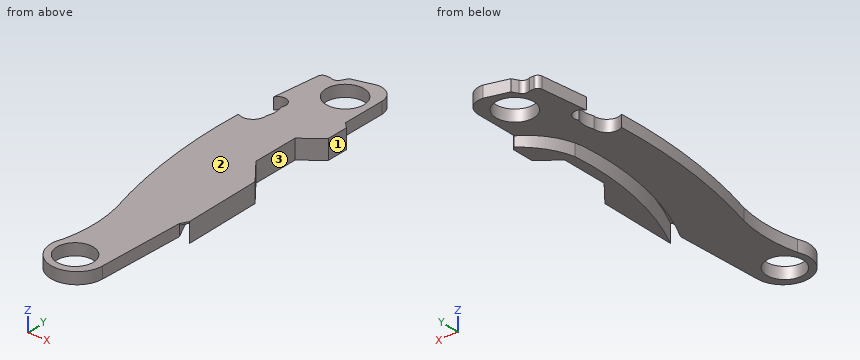
```python
from build123d import *

# Parameters (mm, degrees)
SKETCH1_R           = 3.1115
SKETCH1_R_2         = 2.9845
BOSS_EXTRUDE1_DEPTH = 1.905
CUT_EXTRUDE1_DEPTH  = 1.651
BOSS_EXTRUDE2_START = 1.27
BOSS_EXTRUDE2_DEPTH = 1.27
FILLET1_R           = 0.762
SCALE1_SCALE        = 1.0350841


with BuildPart() as part:
    # Sketch1 → Boss-Extrude1 (new body)
    with BuildSketch(Plane.XY):
        with BuildLine():
            Line((11.455137598, 2.171678291), (10.988691825, -12.194362723))
            ThreePointArc((10.988691825, -12.194362723), (5.753403312, -16.215064409), (2.835732355, -10.293790556))
            ThreePointArc((2.835732355, -10.293790556), (3.433990562, -5.092237988), (2.835732355, 0.109314579))
            ThreePointArc((2.835732355, 0.109314579), (-0.031028462, 13.845472924), (-0.62536344, 27.864999648))
            ThreePointArc((-0.62536344, 27.864999648), (1.430712022, 27.922734075), (2.296539191, 29.788510826))
            ThreePointArc((2.296539191, 29.788510826), (2.577489408, 31.240527695), (2.296539191, 32.692544565))
            ThreePointArc((2.296539191, 32.692544565), (1.793167017, 34.551137871), (-0.054485013, 34.008980516))
            Line((-0.054485013, 34.008980516), (0.8585336, 42.2777508))
            Line((0.8585336, 42.2777508), (2.296539191, 42.2777508))
            ThreePointArc((2.296539191, 42.2777508), (3.056005554, 42.188646363), (3.657600202, 42.660676697))
            Line((3.657600202, 42.660676697), (4.193229273, 43.60832813))
            Line((4.193229273, 43.60832813), (7.858351578, 44.652580854))
            ThreePointArc((7.858351578, 44.652580854), (10.042305559, 44.016121117), (10.988691825, 41.94752521))
            Line((10.988691825, 41.94752521), (10.988691825, 34.921067581))
            Line((10.988691825, 34.921067581), (11.90077889, 34.008980516))
            Line((11.90077889, 34.008980516), (11.90077889, 30.495455397))
            Line((11.90077889, 30.495455397), (8.673783219, 27.864999648))
            Line((8.673783219, 27.864999648), (8.673783219, 20.285030353))
            Line((8.673783219, 20.285030353), (11.90077889, 16.326210266))
            Line((11.90077889, 16.326210266), (12.102967643, 3.372738413))
            Line((12.102967643, 3.372738413), (11.455137598, 2.171678291))
        make_face()
        with Locations(Location((6.72245078, 39.860230894, 0), (0, 0, 180))):
            Circle(SKETCH1_R, mode=Mode.SUBTRACT)
        with Locations(Location((6.525698673, -12.20338788, 0), (0, 0, 180))):
            Circle(SKETCH1_R_2, mode=Mode.SUBTRACT)
    extrude(amount=BOSS_EXTRUDE1_DEPTH)

    # Sketch7 → Cut-Extrude1 (cut)
    with BuildSketch(Plane(origin=(0, 0, 0), x_dir=(-1, 0, 0), z_dir=(0, 0, -1))):
        with BuildLine():
            Line((-12.102967643, 3.372738413), (-11.455137598, 2.171678291))
            ThreePointArc((-11.455137598, 2.171678291), (-6.980280612, 14.413742368), (-6.117233468, 27.41941911))
            ThreePointArc((-6.117233468, 27.41941911), (-7.707175586, 31.719484817), (-10.988691825, 34.921067581))
            Line((-10.988691825, 34.921067581), (-11.444735357, 34.465024049))
            ThreePointArc((-11.444735357, 34.465024049), (-8.702145747, 31.480644967), (-7.139396786, 27.740841235))
            ThreePointArc((-7.139396786, 27.740841235), (-7.956577994, 15.217724405), (-12.102967643, 3.372738413))
        make_face()
    extrude(amount=-CUT_EXTRUDE1_DEPTH, mode=Mode.SUBTRACT)

    # Sketch8 → Boss-Extrude2 (add)
    with BuildSketch(Plane(origin=(0, 0, 0), x_dir=(-1, 0, 0), z_dir=(0, 0, -1)).offset(BOSS_EXTRUDE2_START)):
        with BuildLine():
            Line((-11.90077889, 16.326210266), (-12.102967643, 3.372738413))
            ThreePointArc((-12.102967643, 3.372738413), (-7.956577994, 15.217724405), (-7.139396786, 27.740841235))
            ThreePointArc((-7.139396786, 27.740841235), (-8.702145747, 31.480644967), (-11.444735357, 34.465024049))
            Line((-11.444735357, 34.465024049), (-11.90077889, 34.008980516))
            Line((-11.90077889, 34.008980516), (-11.90077889, 30.495455397))
            Line((-11.90077889, 30.495455397), (-8.673783219, 27.864999648))
            Line((-8.673783219, 27.864999648), (-8.673783219, 20.285030353))
            Line((-8.673783219, 20.285030353), (-11.90077889, 16.326210266))
        make_face()
    extrude(amount=-BOSS_EXTRUDE2_DEPTH)

    # Fillet1
    fillet1_edges = [part.edges().sort_by_distance(p)[0] for p in [
        (0.8585336, 42.2777508, 0.9525),
    ]]
    fillet(fillet1_edges, radius=FILLET1_R)


with BuildPart() as part_1:
    # Scale1: scaled about (6.266812803, 15.225745721, 0.817427893)
    add(part.part.scale(SCALE1_SCALE).moved(Location((-0.219865487, -0.534181585, -0.028678722))))


solid = part_1.part
```
Work out the finished part from the listing and answer in its coordinate system (mm). Face numbers are marked on the shaded views. A direction names the side the tool comes from. Give positions to 0.01 mm unless a question says otherwise; leave off trailing zeros. Order: outer loops, then holes, each group sorted by start corner. A loop starts at its lowest first (then second) coordinate and runs counter-clockwise, first axis right, second up. Notation, with made-up numbers: (34, 18.5) -> (69, 18.5) arc R20 cw to (69, 25.5) -> close; hole circle Ø9 at (-33.5, 6.5). An arc over 180 degrees is marked (long way). Answer as CSV lines item,"result". Start each with the question number.
(1) Section A-A, the plane z = 0.95 is taken. Write down the section's boundary in (x, y) (1 decimal).
(2) Section B-B, the plane x = 5 is taken. Write down the section's boundary in (y, z).
(3) Consider line 1 along Y through (x, z) = (4.5, 1.85); line 2 along X through (y, z) = (24.5, 1.65); line 3 along Y through (x, z) = (5.75, 1.85). Determine where each line is inside the solid, lowest interval first.
(4) Section D-D, the plane y = 4.5 is taken. Write down the section's boundary in (x, z).
(5) Section C-C, the plane y = 41.5 is taken. Write down the section's boundary in (x, z).
(6) Which of the six approach directions +Z, -Z, +X, -X, +Y, -Y give full straight-line access (tool end or side, diameter ignored) to the marked faces 1, 2 and 3?
(7) Each of these flat-tipped pins is pushed along its axis until it touches: pin 1 Ø6.5 at (x, y) = (3, 17.5) entering from -Z; pin 2 Ø1.6 at (y, z) = (39, 0.5) entering from +X; pin 3 Ø0.9 at (x, z) = (1.5, 1) entering from +Y. Where does it stop, or does it pass through?
Entries:
1,outline,"(-0.9, 28.3) arc R89 ccw to (2.7, -0.4) arc R23.7 cw to (2.7, -11.2) arc R4.4 ccw (long way) to (11.2, -13.2) -> (11.6, 1.7) arc R47.6 cw to (6.1, 27.8) arc R10.8 cw to (11.2, 35.6) -> (11.2, 42.9) arc R2.8 ccw to (7.9, 45.7) -> (4.1, 44.6) -> (3.6, 43.6) arc R1 cw to (2.2, 43.2) -> (1.4, 43.2) arc R0.8 ccw to (0.6, 42.5) -> (-0.3, 34.7) arc R1.4 cw (long way) to (2.2, 33.3) arc R4 cw to (2.2, 30.3) arc R2 cw to start; (7.2, 28.2) arc R48 ccw to (12.3, 3) -> (12.1, 16.4) -> (8.8, 20.5) -> (8.8, 28.3) -> (12.1, 31) -> (12.1, 34.7) -> (11.6, 35.1) arc R12.1 ccw to start; hole circle Ø6.2 at (6.5, -13.2); hole circle Ø6.4 at (6.7, 40.7)"
2,outline,"(-17.08, -0.03) -> (-15.85, -0.03) -> (-15.85, 1.94) -> (-17.08, 1.94) -> close; (-10.48, -0.03) -> (38.01, -0.03) -> (38.01, 1.94) -> (-10.48, 1.94) -> close; (43.44, -0.03) -> (44.85, -0.03) -> (44.85, 1.94) -> (43.44, 1.94) -> close"
3,line 1,"-16.82 to -15.49, -10.84 to 38.41, 43.04 to 44.71"
3,line 2,"-0.94 to 5.98, 7.05 to 8.76"
3,line 3,"-17.32 to -16.15, -10.18 to 37.66, 43.79 to 45.07"
4,outline,"(1.41, -0.03) -> (10.26, -0.03) -> (10.26, 1.68) -> (11.55, 1.68) -> (11.55, -1.34) -> (12.28, -1.34) -> (12.28, 1.94) -> (1.41, 1.94) -> close"
5,outline,"(0.48, -0.03) -> (3.61, -0.03) -> (3.61, 1.94) -> (0.48, 1.94) -> close; (9.86, -0.03) -> (11.15, -0.03) -> (11.15, 1.94) -> (9.86, 1.94) -> close"
6,face 1,"+Z, -Z, +X, +Y"
6,face 2,"+Z, +X, -X, +Y, -Y"
6,face 3,"+Z, -Z, +X"
7,pin 1,"z = -0.03"
7,pin 2,"x = 11.15"
7,pin 3,"y = 43.23"
